Design review of the part built by this model. Coordinates are the model's own, in mm. A direction names the side the tool comes from. Give positions to 0.01 mm unless a question says otherwise; leave off trailing zeros. Order: outer loops, then holes, each group sorted by start corner. A loop starts at its lowest first (then second) coordinate and runs counter-clockwise, first axis right, second up. Notation, with made-up numbers: M 89.25,3 L 118.25,3 A18 ccw 118.25,22 Z; hole C 49.5,-10 d1. An arc over 180 degrees is marked long. Answer as a JSON object with one key per item and string values.
from build123d import *

# Parameters (mm, degrees)
SKETCH1_R           = 7.5
BOSS_EXTRUDE1_DEPTH = 320
SKETCH2_R           = 10
BOSS_EXTRUDE2_DEPTH = 5
SKETCH3_R           = 30
BOSS_EXTRUDE3_DEPTH = 5
SKETCH4_R           = 35
SKETCH4_R_2         = 30
BOSS_EXTRUDE4_DEPTH = 30
SKETCH5_R           = 30
BOSS_EXTRUDE5_DEPTH = 5


with BuildPart() as part:
    # Sketch1 → Boss-Extrude1 (new body)
    with BuildSketch(Plane.XY):
        Circle(SKETCH1_R)
    extrude(amount=-BOSS_EXTRUDE1_DEPTH)

    # Sketch2 → Boss-Extrude2 (add)
    with BuildSketch(Plane.XY):
        Circle(SKETCH2_R)
    extrude(amount=BOSS_EXTRUDE2_DEPTH)

    # Sketch3 → Boss-Extrude3 (add)
    with BuildSketch(Plane.XY.offset(5)):
        Circle(SKETCH3_R)
    extrude(amount=BOSS_EXTRUDE3_DEPTH)

    # Sketch4 → Boss-Extrude4 (add)
    # profile 1 of 2: a face of its own
    with BuildSketch(Plane.XY.offset(10)):
        Circle(SKETCH4_R)
        Circle(SKETCH4_R_2, mode=Mode.SUBTRACT)
    # profile 2 of 2: a face of its own
    with BuildSketch(Plane.XY.offset(10)):
        Circle(SKETCH4_R_2)
    extrude(amount=BOSS_EXTRUDE4_DEPTH)

    # Sketch5 → Boss-Extrude5 (add)
    with BuildSketch(Plane.XY.offset(40)):
        Circle(SKETCH5_R)
    extrude(amount=BOSS_EXTRUDE5_DEPTH)


solid = part.part
(1) Tool access review of faces 1 (the flat face through (13, 0, 5)), 2 (the flat face through (0, 0, -320)), 3 (the cylindrical face through (-29.97, 1.32, 42.46)): name each direction out of +Z, -Z, +X, -X, +Y, -Y from which nothing blocks a thin tool from reaching the whole face with its end or side.
Checked values:
{"face 1": "-Z", "face 2": "-Z, +X, -X, +Y, -Y", "face 3": "+Z"}
(2) To check wall thickness, follow L1, parallel to Z at x = 10, y = 12; L2, parallel to Y at x = 0, z = -66.5; L3, parallel to Y at x = -1, z = -262. State the ranges of each line that lie inside material, in increasing order. Write a range as from..to.
Checked values:
{"L1": "z = 5..45", "L2": "y = -7.5..7.5", "L3": "y = -7.43..7.43"}
(3) We need section B-B (x = 0). Write out the cut boundary in (y, z).
Checked values:
{"outline": "M -35,10 L -30,10 L -30,5 L -10,5 L -10,0 L -7.5,0 L -7.5,-320 L 7.5,-320 L 7.5,0 L 10,0 L 10,5 L 30,5 L 30,10 L 35,10 L 35,40 L 30,40 L 30,45 L -30,45 L -30,40 L -35,40 Z"}
(4) We need section A-A (y = 25). Write out the cut boundary in (x, z), plus the area to 3 significant figures.
Checked values:
{"outline": "M -24.49,10 L -16.58,10 L -16.58,5 L 16.58,5 L 16.58,10 L 24.49,10 L 24.49,40 L 16.58,40 L 16.58,45 L -16.58,45 L -16.58,40 L -24.49,40 Z", "area": "1,800 mm^2"}
(5) Insertion check: pin 1 (4 mm diameter, centred on x = 1, z = -38.5, fed in from +Y); pin 2 (2 mm diameter, centred on x = -8, y = -14.5, fed in from -Z). Each pin has a flat end and moves straight along its axis. Give the tip position at first contact, or say it passes through.
Checked values:
{"pin 1": "stops at y = 7.5", "pin 2": "stops at z = 5"}
(6) We need section C-C (z = -12.5). Write out the cut boundary in (x, y), plus the area to 3 significant figures.
Checked values:
{"outline": "C 0,0 d15", "area": "177 mm^2"}
